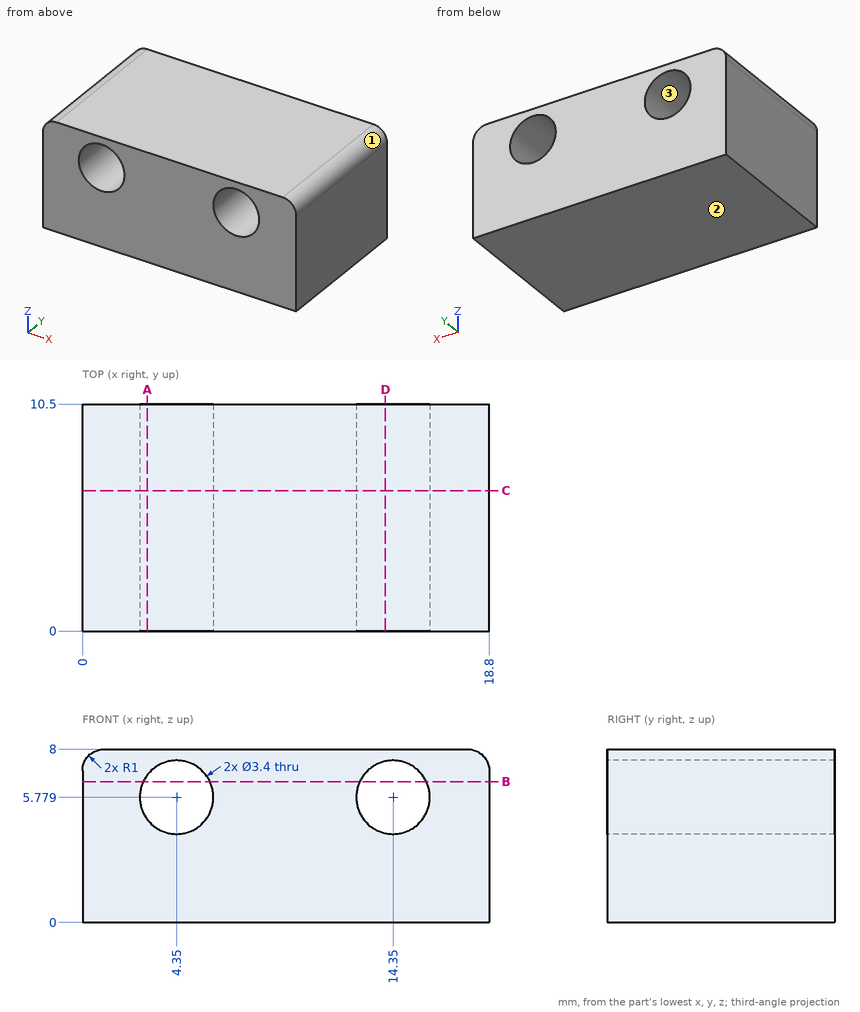
Verification items for this drawing (mm, ordinates from the low corner). Round coordinates to 2 decimals unless told otherwise and drop trailing zeros. Write each loop counter-clockwise with the first axis right and the second up, starting at its lowest first coordinate (ties: lowest second). Pieces come first, ordered by that corner, then holes. Notation, with made-up numbers: (-26.75, 21.5) - (-14.75, 21.5) arc R27 cw to (-14.75, 40.5) - close; hole circle Ø3 at (65, 41). An arc over 180 degrees is marked (long way). One line per item, written item: value.
1. Cross-section at C-C on y = 6.5. Record the boundary of the cut face in (x, z).
The answers:
outline: (0, 0) - (18.8, 0) - (18.8, 7) arc R1 ccw to (17.8, 8) - (1, 8) arc R1 ccw to (0, 7) - close; hole circle Ø3.4 at (4.35, 5.78); hole circle Ø3.4 at (14.35, 5.78)
2. Scan lines: L1, parallel to X at y = 4.25, z = 5.75; L2, parallel to X at y = 7.75, z = 6.5; L3, parallel to Z at x = 4.25, y = 2. Record each from-to range of solid material in increasing order.
The answers:
L1: x = 0 to 2.65, 6.05 to 12.65, 16.05 to 18.8
L2: x = 0 to 2.81, 5.89 to 12.81, 15.89 to 18.8
L3: z = 0 to 4.08, 7.48 to 8
3. Cross-section at A-A on x = 3. Record the boundary of the cut face in (y, z), and give its area (3 significant figures).
The answers:
outline: (0, 0) - (10.5, 0) - (10.5, 4.75) - (0, 4.75) - close; (0, 6.81) - (10.5, 6.81) - (10.5, 8) - (0, 8) - close
area: 62.3 mm^2
4. Cross-section at B-B on z = 6.5. Record the boundary of the cut face in (x, y), and give its area (3 significant figures).
The answers:
outline: (0, 0) - (2.81, 0) - (2.81, 10.5) - (0, 10.5) - close; (5.89, 0) - (12.81, 0) - (12.81, 10.5) - (5.89, 10.5) - close; (15.89, 0) - (18.8, 0) - (18.8, 10.5) - (15.89, 10.5) - close
area: 133 mm^2
5. Mould release check, pull along X, two halves, no side actions. Record for the marked faces 1, 2 and 3: released by +X, released by -X, zero draft, split by the parting line, or undercut.
The answers:
face 1: released by +X
face 2: zero draft
face 3: undercut
6. Cross-section at D-D on x = 14. Record the boundary of the cut face in (y, z).
The answers:
outline: (0, 0) - (10.5, 0) - (10.5, 4.12) - (0, 4.12) - close; (0, 7.44) - (10.5, 7.44) - (10.5, 8) - (0, 8) - close
7. Depth check by flat-ended pin: pin 1 Ø2 at (x, y) = (3, 4.5) entering from -Z. Enter the tip coordinate at first touch or a pass-through.
The answers:
pin 1: stops at z = 0
